The model under review builds one solid part; all positions refer to its coordinate system, in mm. Coordinates: 2 decimals unless noted, no trailing zeros. Write each loop counter-clockwise with the first axis right and the second up, starting at its lowest first coordinate (ties: lowest second). Pieces come first, ordered by that corner, then holes. Notation, with made-up numbers: (25.5, 23.5) - (62.5, 23.5) arc R36 ccw to (62.5, 60.5) - close; hole circle Ø10 at (-10, 87.5). An arc over 180 degrees is marked (long way). Return JSON: item names as keys, results as strings. Group by question number.
(1) We need section A-A on y = 0. State the section outline as (x, z) points, then the cut area to 3 significant figures.
(2) Draft analysis for pull direction Z (two halves, no side actions). For faces 1 (the face through (12, 0, -20)), 2 (the face through (12.325, -3.252, 14.643)), 3 (the face through (12, 20, 74)), state which applies: released by +Z, released by -Z, zero draft, split by the parting line, or undercut.
(3) We need section B-B on x = 12.75. State the section outline as (y, z) points.
(4) We need section D-D on y = -17. State the section outline as (x, z) points.
(5) To check wall thickness, follow L1, parallel to Z at x = 7, y = 0; L2, parallel to Y at x = 20, z = 1; L3, parallel to Z at x = 13, y = 5. State the ranges of each line that lie inside material, in increasing order. Write a range as from..to.
(6) We need section C-C on z = -6. State the section outline as (x, y) points.
(7) For pin 1 Ø3 at (x, y) = (12.5, 12) entering from -Z; pin 2 Ø3 at (x, y) = (16, -9.5) entering from -Z, all flat-tipped, find the tip position at first contact; note any pin that passes through.
```python
from build123d import *

# Parameters (mm, degrees)
F1_DEPTH = 25


with BuildPart() as f1:
    # F0 (on Right) → F1 (new body)
    with BuildSketch(Plane.YZ):
        with BuildLine():
            ThreePointArc((-15, 0), (0, 15), (15, 0))
            Line((15, 0), (20, 0))
            ThreePointArc((20, 0), (0, 20), (-20, 0))
            Line((-20, 0), (-15, 0))
        make_face()
        with BuildLine():
            Line((20, 0), (15, 0))
            ThreePointArc((15, 0), (0, -15), (-15, 0))
            Line((-15, 0), (-20, 0))
            ThreePointArc((-20, 0), (0, -20), (20, 0))
        make_face()
        with BuildLine():
            ThreePointArc((-20, 0), (0, 20), (20, 0))
            Line((20, 0), (20, 150))
            Line((20, 150), (-20, 150))
            Line((-20, 150), (-20, 0))
        make_face()
    extrude(amount=F1_DEPTH)


solid = f1.part
```
Ans:
{
 "1": {"outline": "(0, -20) - (25, -20) - (25, -15) - (0, -15) - close; (0, 15) - (25, 15) - (25, 150) - (0, 150) - close", "area": "3,500 mm²"},
 "2": {"face 1": "released by -Z", "face 2": "undercut", "face 3": "zero draft"},
 "3": {"outline": "(-20, 0) arc R20 ccw to (20, 0) - (20, 150) - (-20, 150) - close; hole circle Ø30 at (0, 0)"},
 "4": {"outline": "(0, -10.54) - (25, -10.54) - (25, 150) - (0, 150) - close"},
 "5": {"L1": "-20..-15, 15..150", "L2": "-20..-14.97, 14.97..20", "L3": "-19.36..-14.14, 14.14..150"},
 "6": {"outline": "(0, -19.08) - (25, -19.08) - (25, -13.75) - (0, -13.75) - close; (0, 13.75) - (25, 13.75) - (25, 19.08) - (0, 19.08) - close"},
 "7": {"pin 1": "z = -17.02", "pin 2": "z = -18.33"}
}
